Input: part model. Units: mm. Frame: model coordinates. Face numbers are marked on the shaded views. Give positions to 0.01 mm unless a question says otherwise; leave off trailing zeros. Order: outer loops, then holes, each group sorted by start corner. A loop starts at its lowest first (then second) coordinate and runs counter-clockwise, first axis right, second up.
```python
from build123d import *

# Parameters (mm, degrees)
FLANGE_BASE2_DEPTH       = 137.5
CORTE_EXTRUS_O3_START    = -137.5
CORTE_EXTRUS_O3_DEPTH    = 13
CORTE_EXTRUS_O3_START_2  = 124.5
CORTE_EXTRUS_O3_2_DEPTH  = 13
ESBO_O12_W               = 13
ESBO_O12_H               = 1.2
RESSALTO_EXTRUS_O1_DEPTH = 19
FILETE1_R                = 1
ESBO_O13_R               = 5
CORTE_EXTRUS_O4_DEPTH    = 140.208225332


# Read off the part's stored shape, not the designer's step: Corte-extrusão3
# Sheet-metal steps are written as plain solids
with BuildPart() as part:
    # Esboço1 → Flange-base2 (new, symmetric)
    with BuildSketch(Plane(origin=(0, 0, 0), x_dir=(0, 0, -1), z_dir=(1, 0, 0))):
        with BuildLine():
            Line((-18, 9), (-18, 0.7366))
            ThreePointArc((-18, 0.7366), (-17.784254855, 0.215745145), (-17.2634, 0))
            Line((-17.2634, 0), (17.2634, 0))
            ThreePointArc((17.2634, 0), (17.784254855, 0.215745145), (18, 0.7366))
            Line((18, 0.7366), (18, 3))
            Line((18, 3), (19.2, 3))
            Line((19.2, 3), (19.2, 0.7366))
            ThreePointArc((19.2, 0.7366), (18.632782992, -0.632782992), (17.2634, -1.2))
            Line((17.2634, -1.2), (-17.2634, -1.2))
            ThreePointArc((-17.2634, -1.2), (-18.632782992, -0.632782992), (-19.2, 0.7366))
            Line((-19.2, 0.7366), (-19.2, 9))
            Line((-19.2, 9), (-18, 9))
        make_face()
    extrude(amount=FLANGE_BASE2_DEPTH, both=True)

    # Corte-extrusão3 outline → Corte-extrusão3 (cut)
    with BuildSketch(Plane.YZ.offset(CORTE_EXTRUS_O3_START)):
        with BuildLine():
            Line((-1.2, 17.2634), (0, 17.2634))
            ThreePointArc((0, 17.2634), (0.215745145, 17.784254855), (0.7366, 18))
            Line((0.7366, 18), (9, 18))
            Line((9, 18), (9, 19.2))
            Line((9, 19.2), (0.7366, 19.2))
            ThreePointArc((0.7366, 19.2), (-0.632782992, 18.632782992), (-1.2, 17.2634))
        make_face()
        with BuildLine():
            ThreePointArc((0.7366, -18), (0.215745145, -17.784254855), (0, -17.2634))
            Line((0, -17.2634), (-1.2, -17.2634))
            ThreePointArc((-1.2, -17.2634), (-0.632782992, -18.632782992), (0.7366, -19.2))
            Line((0.7366, -19.2), (3, -19.2))
            Line((3, -19.2), (3, -18))
            Line((3, -18), (0.7366, -18))
        make_face()
    extrude(amount=CORTE_EXTRUS_O3_DEPTH, mode=Mode.SUBTRACT)

    # Corte-extrus_o3 2 outline → Corte-extrus_o3 2 (cut)
    with BuildSketch(Plane.YZ.offset(CORTE_EXTRUS_O3_START_2)):
        with BuildLine():
            Line((-1.2, 17.2634), (0, 17.2634))
            ThreePointArc((0, 17.2634), (0.215745145, 17.784254855), (0.7366, 18))
            Line((0.7366, 18), (9, 18))
            Line((9, 18), (9, 19.2))
            Line((9, 19.2), (0.7366, 19.2))
            ThreePointArc((0.7366, 19.2), (-0.632782992, 18.632782992), (-1.2, 17.2634))
        make_face()
        with BuildLine():
            ThreePointArc((0.7366, -18), (0.215745145, -17.784254855), (0, -17.2634))
            Line((0, -17.2634), (-1.2, -17.2634))
            ThreePointArc((-1.2, -17.2634), (-0.632782992, -18.632782992), (0.7366, -19.2))
            Line((0.7366, -19.2), (3, -19.2))
            Line((3, -19.2), (3, -18))
            Line((3, -18), (0.7366, -18))
        make_face()
    extrude(amount=CORTE_EXTRUS_O3_2_DEPTH, mode=Mode.SUBTRACT)

    # Esboço12 → Ressalto-extrusão1 (add, symmetric)
    with BuildSketch(Plane.XY):
        with Locations((131, -0.6)):
            Rectangle(ESBO_O12_W, ESBO_O12_H)
        with Locations((-131, -0.6)):
            Rectangle(ESBO_O12_W, ESBO_O12_H)
    extrude(amount=RESSALTO_EXTRUS_O1_DEPTH, both=True)

    # Filete1
    filete1_edges = [part.edges().sort_by_distance(p)[0] for p in [
        (137.5, -0.6, -19),
        (137.5, -0.6, 19),
        (-137.5, -0.6, -19),
        (-137.5, -0.6, 19),
    ]]
    fillet(filete1_edges, radius=FILETE1_R)

    # Esboço13 → Corte-extrusão4 (cut, through all)
    with BuildSketch(Plane.XZ.offset(1.2)):
        with Locations(Location((87.5, 9.2, 0), (0, 0, 270))):
            Circle(ESBO_O13_R)
    extrude(amount=-CORTE_EXTRUS_O4_DEPTH, mode=Mode.SUBTRACT)


solid = part.part
```
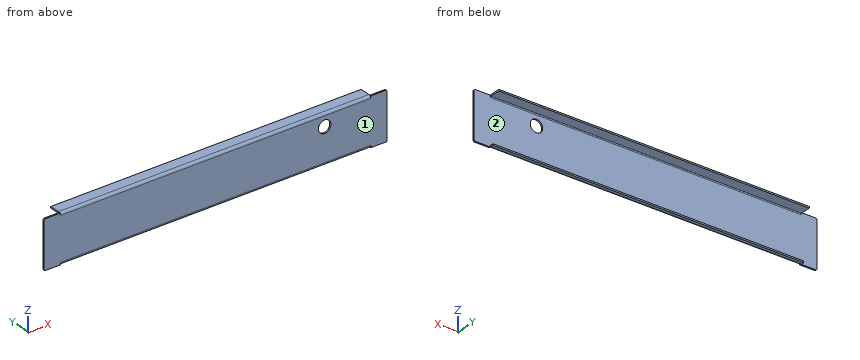
1) First-contact query: P1, Ø0.6, axis at y = 2, z = -18.5, coming from the -X side; P2, Ø1.5, axis at x = 5.5, z = -7, coming from the +Y side; P3, Ø1.5, axis at y = 1, z = -18, coming from the +X side; P4, Ø2.5, axis at x = 6, y = 4, coming from the -Z side. Flat tips, straight axial feed; report the tip coordinate or a pass-through.
2) Line query: probe 1 along Z at (x, y) = (69, 1.5); probe 2 along X at (y, z) = (-0.85, 9.2); probe 3 along Y at (x, z) = (59, 0). Output: solid intervals per line, ascending.
3) Cut plane A-A (z = 9.2). Return the cut outline in (x, y), then the cut area to 3 significant figures.
4) Pull-direction query (Z, two-part tool) for the marked faces 1 and 2; classes: pulls with the +Z half, pulls with the -Z half, needs draft (parallel to the pull), parting line crosses it, or undercut.
5) Cut plane B-B (x = 87.5). Return the cut outline in (y, z).
6) Cut plane C-C (x = -107.5). Return the cut outline in (y, z), then the cut area to 3 significant figures.
7) Cut plane D-D (z = -14). Return the cut outline in (x, y), then the cut area to 3 significant figures.
Geometry says:
1. P1: stops at x = -124.5
1. P2: stops at y = 0
1. P3: stops at x = 124.5
1. P4: stops at z = -19.2
2. probe 1: z = -19.2 to -18, 18 to 19.2
2. probe 2: x = -137.5 to 82.5, 92.5 to 137.5
2. probe 3: y = -1.2 to 0
3. outline: (-137.5, -1.2) - (82.5, -1.2) - (82.5, 0) - (-137.5, 0) - close; (92.5, -1.2) - (137.5, -1.2) - (137.5, 0) - (92.5, 0) - close
3. area: 318 mm2
4. face 1: needs draft
4. face 2: undercut
5. outline: (-1.2, -17.26) arc R1.94 ccw to (0.74, -19.2) - (3, -19.2) - (3, -18) - (0.74, -18) arc R0.74 cw to (0, -17.26) - (0, 4.2) - (-1.2, 4.2) - close; (-1.2, 14.2) - (0, 14.2) - (0, 17.26) arc R0.74 cw to (0.74, 18) - (9, 18) - (9, 19.2) - (0.74, 19.2) arc R1.94 ccw to (-1.2, 17.26) - close
6. outline: (-1.2, -17.26) arc R1.94 ccw to (0.74, -19.2) - (3, -19.2) - (3, -18) - (0.74, -18) arc R0.74 cw to (0, -17.26) - (0, 17.26) arc R0.74 cw to (0.74, 18) - (9, 18) - (9, 19.2) - (0.74, 19.2) arc R1.94 ccw to (-1.2, 17.26) - close
6. area: 59.1 mm2
7. outline: (-137.5, -1.2) - (137.5, -1.2) - (137.5, 0) - (-137.5, 0) - close
7. area: 330 mm2
